```python
from build123d import *

# Parameters (mm, degrees)
F0_R     = 2.5
F1_DEPTH = 7.5


with BuildPart() as f1:
    # F0 (on Front) → F1 (new body, symmetric)
    with BuildSketch(Plane.XZ):
        Polygon((-667.819926, 0), (0, 0), (0, 200), (-703.085322, 200), align=None)
        with Locations((-642.646937, 30)):
            Circle(F0_R, mode=Mode.SUBTRACT)
        with Locations((-500.487212, 30)):
            Circle(F0_R, mode=Mode.SUBTRACT)
        with Locations((-170, 30)):
            Circle(F0_R, mode=Mode.SUBTRACT)
        with Locations((-30, 30)):
            Circle(F0_R, mode=Mode.SUBTRACT)
        with Locations((-667.332715, 170)):
            Circle(F0_R, mode=Mode.SUBTRACT)
        with Locations((-525.172989, 170)):
            Circle(F0_R, mode=Mode.SUBTRACT)
        with Locations((-170, 170)):
            Circle(F0_R, mode=Mode.SUBTRACT)
        with Locations((-30, 170)):
            Circle(F0_R, mode=Mode.SUBTRACT)
    extrude(amount=F1_DEPTH, both=True)


solid = f1.part
```
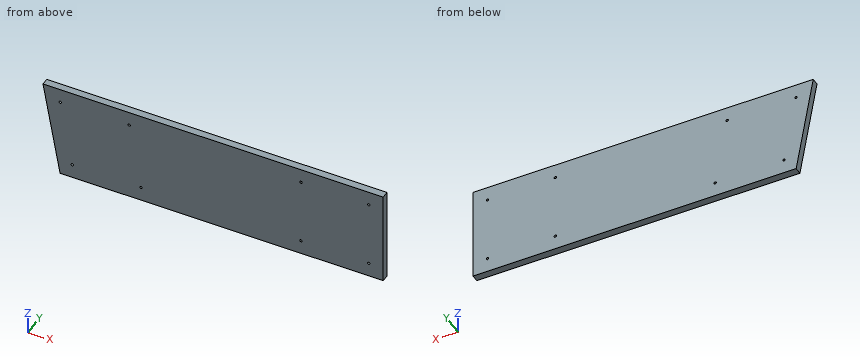
The model under review builds one solid part; all positions refer to its coordinate system, in mm. Give positions to 0.01 mm unless a question says otherwise; leave off trailing zeros. Write each loop counter-clockwise with the first axis right and the second up, starting at its lowest first coordinate (ties: lowest second). Pieces come first, ordered by that corner, then holes. Notation, with made-up numbers: M 70.25,46.5 L 103.25,46.5 A11 cw 103.25,66.5 Z; hole C 23.5,59.5 d4. An arc over 180 degrees is marked long. Write each question's results on one line, items separated by ' | '. Start each with the question number.
1. We need section B-B (z = 107.5). Write out the cut boundary in (x, y), and give its area (3 significant figures).
2. We need section C-C (z = 69). Write out the cut boundary in (x, y).
3. We need section A-A (y = 4.75). Count the separate pieces of the cut face and the enclosed holes in it, and give its area (3 significant figures).
4. For probe 1 along Z at (x, y) = (-170, 0.75); probe 2 along X at (y, z) = (2.75, 170); probe 3 along Z at (x, y) = (-642.5, 4.5), list the stretches that pass through material, from the lowest coordinate up. Write a range as [from, to].
Results found:
1) outline: M -686.78,-7.5 L 0,-7.5 L 0,7.5 L -686.78,7.5 Z | area: 10,300 mm^2
2) outline: M -679.99,-7.5 L 0,-7.5 L 0,7.5 L -679.99,7.5 Z
3) separate pieces: 1 | enclosed holes: 8 | area: 137,000 mm^2
4) probe 1: z = [0, 27.5], [32.5, 167.5], [172.5, 200] | probe 2: x = [-697.8, -669.83], [-664.83, -527.67], [-522.67, -172.5], [-167.5, -32.5], [-27.5, 0] | probe 3: z = [0, 27.5], [32.5, 200]
